Geometry check sheet. Reference: the model listing, model coordinates, mm. A direction names the side the tool comes from. Round coordinates to 2 decimals unless told otherwise and drop trailing zeros. Order: outer loops, then holes, each group sorted by start corner. A loop starts at its lowest first (then second) coordinate and runs counter-clockwise, first axis right, second up.
```python
from build123d import *

# Parameters (mm, degrees)
SKETCH1_R           = 1
BOSS_EXTRUDE1_DEPTH = 4.7


with BuildPart() as part:
    # Sketch1 → Boss-Extrude1 (new body)
    with BuildSketch(Plane.XY):
        Polygon((0, 3.85), (0.623058615, 2.729798154), (1.670452396, 3.468730141), (1.745771445, 2.189128151), (3.010051208, 2.400435737), (2.52271283, 1.21487447), (3.753472462, 0.856705596), (2.8, 0), (3.753472462, -0.856705596), (2.52271283, -1.21487447), (3.010051208, -2.400435737), (1.745771445, -2.189128151), (1.670452396, -3.468730141), (0.623058615, -2.729798154), (0, -3.85), (-0.623058615, -2.729798154), (-1.670452396, -3.468730141), (-1.745771445, -2.189128151), (-3.010051208, -2.400435737), (-2.52271283, -1.21487447), (-3.753472462, -0.856705596), (-2.8, 0), (-3.753472462, 0.856705596), (-2.52271283, 1.21487447), (-3.010051208, 2.400435737), (-1.745771445, 2.189128151), (-1.670452396, 3.468730141), (-0.623058615, 2.729798154), align=None)
        Circle(SKETCH1_R, mode=Mode.SUBTRACT)
    extrude(amount=BOSS_EXTRUDE1_DEPTH)


solid = part.part
```
(1) Draft check along X on faces 1 (the flat face through (-2.4, -2.3, 2.3)), 2 (the flat face through (-2.77, -1.82, 2.32)), 3 (the flat face through (3.27, -0.42, 2.32)). Enter one of: released by +X, released by -X, zero draft, split by the parting line, or undercut.
Returned:
face 1: undercut
face 2: released by -X
face 3: released by +X
(2) Material ranges on line 1 (X direction, y = -3, z = 1.95); line 2 (Y direction, x = 2.75, z = 2.7); line 3 (Y direction, x = -0.5, z = 0.2), recorded low to high.
Returned:
line 1: x = -1.7 to -1.01, -0.47 to 0.47, 1.01 to 1.7
line 2: y = -2.36 to -1.77, -1.15 to 1.15, 1.77 to 2.36
line 3: y = -2.95 to -0.87, 0.87 to 2.95
(3) Set-up check for faces 4 (the flat face through (3.13, 1.04, 2.32)), 5 (the flat face through (-1.15, 3.1, 2.32)), 6 (the flat face through (2.4, -2.3, 2.3)): record each of +Z, -Z, +X, -X, +Y, -Y from which the full face is reachable in a straight line by a thin tool's end or side.
Returned:
face 4: +Z, -Z, +X
face 5: +Z, -Z, +Y
face 6: +Z, -Z, -Y
(4) Depth check by flat-ended pin: P1, Ø1, axis at y = 2.5, z = 4, coming from the +X side; P2, Ø2, axis at y = 0, z = 2.5, coming from the +X side. Enter the tip coordinate at first touch or a pass-through.
Returned:
P1: stops at x = 3.01
P2: stops at x = 3.75
(5) Sectioned sample at C-C, the plane y = 3.25. Record the cut outline in (x, z).
Returned:
outline: (-1.68, 0) - (-1.36, 0) - (-1.36, 4.7) - (-1.68, 4.7) - close; (-0.33, 0) - (0.33, 0) - (0.33, 4.7) - (-0.33, 4.7) - close; (1.36, 0) - (1.68, 0) - (1.68, 4.7) - (1.36, 4.7) - close
(6) Sectioned sample at B-B, the plane y = 0.5. Record the cut outline in (x, z), and give its area (3 significant figures).
Returned:
outline: (-3.36, 0) - (-0.87, 0) - (-0.87, 4.7) - (-3.36, 4.7) - close; (0.87, 0) - (3.36, 0) - (3.36, 4.7) - (0.87, 4.7) - close
area: 23.4 mm2
(7) Sectioned sample at D-D, the plane x = -1.25. Record the cut outline in (y, z).
Returned:
outline: (-3.17, 0) - (3.17, 0) - (3.17, 4.7) - (-3.17, 4.7) - close
